from build123d import *

# Parameters (mm, degrees)
F1_DEPTH = 250
F4_DEPTH = 25
F5_R     = 25.0490469986
F6_DEPTH = 200


with BuildPart() as f1:
    # F0 (on Front) → F1 (new body)
    with BuildSketch(Plane.XZ):
        with BuildLine():
            ThreePointArc((53.7174828351, 43.0048087239), (50.7885506469, 50.0758765358), (43.7174828351, 53.0048087239))
            Line((43.7174828351, 53.0048087239), (-43.7174828351, 53.0048087239))
            ThreePointArc((-43.7174828351, 53.0048087239), (-50.7885506469, 50.0758765358), (-53.7174828351, 43.0048087239))
            Line((-53.7174828351, 43.0048087239), (-53.7174828351, -43.0048087239))
            ThreePointArc((-53.7174828351, -43.0048087239), (-50.7885506469, -50.0758765358), (-43.7174828351, -53.0048087239))
            Line((-43.7174828351, -53.0048087239), (43.7174828351, -53.0048087239))
            ThreePointArc((43.7174828351, -53.0048087239), (50.7885506469, -50.0758765358), (53.7174828351, -43.0048087239))
            Line((53.7174828351, -43.0048087239), (53.7174828351, 43.0048087239))
        make_face()
    extrude(amount=F1_DEPTH)

    # F2 (on face) + F3 (on face) → F4 (join)
    with BuildSketch(Plane.XZ.offset(250)):
        with BuildLine():
            Line((-60.7174821198, 43.0048087239), (-60.7174821198, -43.0048087239))
            ThreePointArc((-60.7174821198, -43.0048087239), (-55.7382976095, -55.0256234983), (-43.7174828351, -60.0048080087))
            Line((-43.7174828351, -60.0048080087), (43.7174828351, -60.0048080087))
            ThreePointArc((43.7174828351, -60.0048080087), (55.7382976095, -55.0256234983), (60.7174821198, -43.0048087239))
            Line((60.7174821198, -43.0048087239), (60.7174821198, 43.0048087239))
            ThreePointArc((60.7174821198, 43.0048087239), (55.7382976095, 55.0256234983), (43.7174828351, 60.0048080087))
            Line((43.7174828351, 60.0048080087), (-43.7174828351, 60.0048080087))
            ThreePointArc((-43.7174828351, 60.0048080087), (-55.7382976095, 55.0256234983), (-60.7174821198, 43.0048087239))
        make_face()
    with BuildSketch(Plane(origin=(0, 0, 0), x_dir=(-1, 0, 0), z_dir=(0, 1, 0))):
        with BuildLine():
            Line((-60.7174821198, 43.0048087239), (-60.7174821198, -43.0048087239))
            ThreePointArc((-60.7174821198, -43.0048087239), (-55.7382976095, -55.0256234983), (-43.7174828351, -60.0048080087))
            Line((-43.7174828351, -60.0048080087), (43.7174828351, -60.0048080087))
            ThreePointArc((43.7174828351, -60.0048080087), (55.7382976095, -55.0256234983), (60.7174821198, -43.0048087239))
            Line((60.7174821198, -43.0048087239), (60.7174821198, 43.0048087239))
            ThreePointArc((60.7174821198, 43.0048087239), (55.7382976095, 55.0256234983), (43.7174828351, 60.0048080087))
            Line((43.7174828351, 60.0048080087), (-43.7174828351, 60.0048080087))
            ThreePointArc((-43.7174828351, 60.0048080087), (-55.7382976095, 55.0256234983), (-60.7174821198, 43.0048087239))
        make_face()
    extrude(amount=F4_DEPTH, dir=(0, -1, 0))

    # F5 (on face) → F6 (join)
    with BuildSketch(Plane(origin=(0, 0, 0), x_dir=(-1, 0, 0), z_dir=(0, 1, 0))):
        Circle(F5_R)
    extrude(amount=F6_DEPTH)


solid = f1.part
The listing builds one solid part. Answer for the finished solid, in the listing's coordinates (mm). A direction names the side the tool comes from. Round coordinates to 2 decimals unless told otherwise and drop trailing zeros. Write each loop counter-clockwise with the first axis right and the second up, starting at its lowest first coordinate (ties: lowest second). Pieces come first, ordered by that corner, then holes. Notation, with made-up numbers: M -18,7.5 L 17,7.5 A29 cw 17,34.5 Z; hole C 13.5,-20.75 d5. An arc over 180 degrees is marked long. Write each question's results on one line, items separated by ' | '. Start each with the question number.
Item 1: For faces 5 (the face through (1, -136, 53.005)), 6 (the face through (-53.717, -136, 1)), 7 (the face through (-23.9, 98.6, 7.5)), determine the directions among +Z, -Z, +X, -X, +Y, -Y from which every point of the face is accessible in a straight line to the end or side of a thin tool.
Item 2: For a pull along Y with two mould halves and no side action, classify faces 1 (the face through (50.71, -135.925, -50.153)), 2 (the face through (-1, -275, 1)), 3 (the face through (0, 200, 0)), 4 (the face through (-60.717, -262, 1)) as pulls with the +Y half, pulls with the -Y half, needs draft (parallel to the pull), parting line crosses it, or undercut.
Item 3: A cutting plane is placed at A-A on z = -32. Write down the section's boundary in (x, y).
Item 4: A cutting plane is placed at C-C on y = -149. Write down the section's boundary in (x, z), and give its area (3 significant figures).
Item 5: Straight lines are drawn through the part: L1, parallel to Y at x = 28, z = -54.5; L2, parallel to Z at x = 19, y = -130; L3, parallel to X at y = -143, z = 3.5. For each, find the intervals that lie inside material, in ascending order. Write a range as [from, to].
Item 6: A cutting plane is placed at B-B on x = 0. Write down the section's boundary in (y, z).
Item 7: A cutting plane is placed at D-D on z = -7. Write down the section's boundary in (x, y), and give its area (3 significant figures).
Item 8: Flat-ended cylindrical pins translate along their axes: pin 1 Ø1 at (x, y) = (-1, 37.5) entering from -Z; pin 2 Ø5 at (y, z) = (37.5, 1) entering from +X; pin 3 Ø1.5 at (x, z) = (-30.5, 25.5) entering from +Y. Find the tip coordinate at first contact, or state that the pin passes through.
Check sheet entries:
1) face 5: +Z, +X, -X | face 6: +Z, -Z, -X | face 7: +Y
2) face 1: undercut | face 2: pulls with the -Y half | face 3: pulls with the +Y half | face 4: needs draft
3) outline: M -60.72,-275 L 60.72,-275 L 60.72,-250 L 53.72,-250 L 53.72,-25 L 60.72,-25 L 60.72,0 L -60.72,0 L -60.72,-25 L -53.72,-25 L -53.72,-250 L -60.72,-250 Z
4) outline: M -53.72,-43 A10 ccw -43.72,-53 L 43.72,-53 A10 ccw 53.72,-43 L 53.72,43 A10 ccw 43.72,53 L -43.72,53 A10 ccw -53.72,43 Z | area: 11,300 mm²
5) L1: [-275, -250], [-25, 0] | L2: [-53, 53] | L3: [-53.72, 53.72]
6) outline: M -275,-60 L -250,-60 L -250,-53 L -25,-53 L -25,-60 L 0,-60 L 0,-25.05 L 200,-25.05 L 200,25.05 L 0,25.05 L 0,60 L -25,60 L -25,53 L -250,53 L -250,60 L -275,60 Z
7) outline: M -60.72,-275 L 60.72,-275 L 60.72,-250 L 53.72,-250 L 53.72,-25 L 60.72,-25 L 60.72,0 L 24.05,0 L 24.05,200 L -24.05,200 L -24.05,0 L -60.72,0 L -60.72,-25 L -53.72,-25 L -53.72,-250 L -60.72,-250 Z | area: 39,900 mm²
8) pin 1: z = -25.04 | pin 2: x = 25.05 | pin 3: y = 0
